The listing builds one solid part. Answer for the finished solid, in the listing's coordinates (mm). A direction names the side the tool comes from. Coordinates: 2 decimals unless noted, no trailing zeros. Order: outer loops, then holes, each group sorted by start corner. A loop starts at its lowest first (then second) coordinate and runs counter-clockwise, first axis right, second up. Notation, with made-up numbers: (-12, 52) -> (27, 52) arc R29 cw to (27, 72) -> close; hole circle Ø9 at (-30, 37). An arc over 180 degrees is marked (long way). Write each question's results on one line, items separated by ' | '. Start each with the question number.
(1) The part is cut by section A-A, the plane z = -5. Give the vertices of the cut face in (x, y), then the cut area to 3 significant figures.
(2) A tool of negligible diameter and unlimited length cuts with its end or side. For faces 1 (the face through (0, 2, 20.5)), 2 (the face through (40, 2, 0)), 3 (the face through (-40, 2, 0)), from which of +Z, -Z, +X, -X, +Y, -Y can it reach the whole face along a straight path? Write none if from no direction.
(3) Straight lines are drawn through the part: L1, parallel to X at y = 3.3, z = 16.25; L2, parallel to X at y = 1, z = 33.5; L3, parallel to Z at x = 40, y = 3.75. For each, find the intervals that lie inside material, in ascending order.
(4) The part is cut by section B-B, the plane x = -7.5. Give the vertices of the cut face in (y, z).
(5) Given pin 1 (4 mm diameter, centred on x = -31, z = 33.5, fed in from -Y); pin 2 (1.4 mm diameter, centred on y = 2, z = -6.5, fed in from +X), each flat-ended and moving along its own axis, determine where each tip first touches the part or whether it passes through.
(6) The part is cut by section C-C, the plane y = 0.9. Count the separate pieces of the cut face and the enclosed holes in it, then the cut area to 3 significant figures.
(7) The part is cut by section D-D, the plane z = 33.5. Give the vertices of the cut face in (x, y).
(8) Determine the mould class of faces 4 (the face through (-1, 0, 29)), 5 (the face through (-21.5, 2, 16)), 6 (the face through (21.5, 2, 16)), 7 (the face through (45, 2, 35)) for opening direction X: +X half, -X half, draft (parallel to the pull), parting line (faces both ways), or undercut.
```python
from build123d import *

# Parameters (mm, degrees)
BASE_DEPTH         = 4.7625
SKETCH2_R          = 1.5625
CUT_EXTRUDE1_DEPTH = 5.7625
SKETCH3_R          = 2.286
SKETCH3_W          = 43
SKETCH3_H          = 8.5
CUT_EXTRUDE2_DEPTH = 5.7625
SKETCH4_R          = 1.45
CUT_EXTRUDE3_DEPTH = 5.7625
SKETCH5_R          = 0.5
CUT_EXTRUDE4_DEPTH = 5.7625


with BuildPart() as part:
    # Sketch1 → Base (new body)
    with BuildSketch(Plane(origin=(0, 0, 0), x_dir=(1, 0, 0), z_dir=(0, 1, 0))):
        Polygon((-35, 0), (-45, 0), (-45, -70), (45, -70), (45, 0), (35, 0), (35, 10), (-35, 10), align=None)
    extrude(amount=BASE_DEPTH)

    # Sketch2 → Cut-Extrude1 (cut, through all)
    with BuildSketch(Plane(origin=(0, 4.7625, 0), x_dir=(1, 0, 0), z_dir=(0, 1, 0))):
        with Locations((-31, -33.5)):
            Circle(SKETCH2_R)
        with Locations((0, -33.5)):
            Circle(SKETCH2_R)
        with Locations((31, -33.5)):
            Circle(SKETCH2_R)
        with Locations((15, -49.5)):
            Circle(SKETCH2_R)
        with Locations((-15, -49.5)):
            Circle(SKETCH2_R)
    extrude(amount=-CUT_EXTRUDE1_DEPTH, mode=Mode.SUBTRACT)

    # Sketch3 → Cut-Extrude2 (cut, through all)
    with BuildSketch(Plane(origin=(0, 4.7625, 0), x_dir=(1, 0, 0), z_dir=(0, 1, 0))):
        with Locations((-26, -16.25)):
            Circle(SKETCH3_R)
        with Locations((26, -16.25)):
            Circle(SKETCH3_R)
        with Locations((0, -16.25)):
            Rectangle(SKETCH3_W, SKETCH3_H)
    extrude(amount=-CUT_EXTRUDE2_DEPTH, mode=Mode.SUBTRACT)

    # Sketch4 → Cut-Extrude3 (cut, through all)
    with BuildSketch(Plane(origin=(0, 4.7625, 0), x_dir=(1, 0, 0), z_dir=(0, 1, 0))):
        with Locations((-28, 5)):
            Circle(SKETCH4_R)
        with Locations((-40, -7)):
            Circle(SKETCH4_R)
        with Locations((-40, -63)):
            Circle(SKETCH4_R)
        with Locations((40, -63)):
            Circle(SKETCH4_R)
        with Locations((40, -7)):
            Circle(SKETCH4_R)
        with Locations((28, 5)):
            Circle(SKETCH4_R)
    extrude(amount=-CUT_EXTRUDE3_DEPTH, mode=Mode.SUBTRACT)

    # Sketch5 → Cut-Extrude4 (cut, through all)
    with BuildSketch(Plane(origin=(0, 4.7625, 0), x_dir=(1, 0, 0), z_dir=(0, 1, 0))):
        with Locations((-35.25, 0.25)):
            Circle(SKETCH5_R)
        with Locations((-21.25, -12.25)):
            Circle(SKETCH5_R)
        with Locations((-21.25, -20.25)):
            Circle(SKETCH5_R)
        with Locations((35.25, 0.25)):
            Circle(SKETCH5_R)
        with Locations((21.25, -12.25)):
            Circle(SKETCH5_R)
        with Locations((21.25, -20.25)):
            Circle(SKETCH5_R)
    extrude(amount=-CUT_EXTRUDE4_DEPTH, mode=Mode.SUBTRACT)


solid = part.part
```
Established:
1) outline: (-35, 0) -> (-29.45, 0) -> (-29.45, 4.76) -> (-35, 4.76) -> close; (-26.55, 0) -> (26.55, 0) -> (26.55, 4.76) -> (-26.55, 4.76) -> close; (29.45, 0) -> (35, 0) -> (35, 4.76) -> (29.45, 4.76) -> close | area: 306 mm^2
2) face 1: +Y, -Y | face 2: -Z, +X, +Y, -Y | face 3: -Z, -X, +Y, -Y
3) L1: x = -45 to -28.29, -23.71 to -21.5, 21.5 to 23.71, 28.29 to 45 | L2: x = -45 to -32.56, -29.44 to -1.56, 1.56 to 29.44, 32.56 to 45 | L3: z = 0 to 5.55, 8.45 to 61.55, 64.45 to 70
4) outline: (0, -10) -> (4.76, -10) -> (4.76, 12) -> (0, 12) -> close; (0, 20.5) -> (4.76, 20.5) -> (4.76, 70) -> (0, 70) -> close
5) pin 1: stops at y = 0 | pin 2: stops at x = 35
6) separate pieces: 1 | enclosed holes: 14 | area: 6,520 mm^2
7) outline: (-45, 0) -> (-32.56, 0) -> (-32.56, 4.76) -> (-45, 4.76) -> close; (-29.44, 0) -> (-1.56, 0) -> (-1.56, 4.76) -> (-29.44, 4.76) -> close; (1.56, 0) -> (29.44, 0) -> (29.44, 4.76) -> (1.56, 4.76) -> close; (32.56, 0) -> (45, 0) -> (45, 4.76) -> (32.56, 4.76) -> close
8) face 4: draft | face 5: undercut | face 6: undercut | face 7: +X half
